Here's how the part is built. I have some questions about the finished solid (model axes, mm). A direction names the side the tool comes from. Give positions to 0.01 mm unless a question says otherwise; leave off trailing zeros. Loops run counter-clockwise (first coordinate to the right, second up) from the corner with the lowest first, then second, coordinate; pieces in that order, holes last.
Q1. Suppose I cut it at B-B (z = 27.5). List the corners of the cut face in (x, y) for me.
Q2. Suppose I cut it at D-D (y = -57). List the corners of the cut face in (x, z) for me.
Q3. I'm going to push flat-ended pins straight in: P1, Ø6, axis at x = 28.5, y = -5.5, coming from the -Z side; P2, Ø9, axis at y = 0, z = 0, coming from the -X side. Where does each tip first touch, or does it pass through?
Q4. For faces 5 (the face through (0, 7, 0)), 6 (the face through (5, 15, 0)), which set-ups out of +Z, -Z, +X, -X, +Y, -Y let a thin tool reach every point of the face, with its end or its side?
Q5. Suppose I cut it at A-A (y = 0). List the corners of the cut face in (x, z) for me.
Q6. I need wall thicknesses on probe 1 along X at (y, z) = (-14, -4); probe 2 along Y at (x, z) = (12.5, 0); probe 3 along Y at (x, z) = (38, 1.5). Which ranges of each line are inside material? Lowest first, please.
Q7. Suppose I cut it at C-C (x = 42.5). List the corners of the cut face in (y, z) for me, and give its area (3 significant figures).
Q8. Thinking about a two-plate mould opening in X: for faces 1 (the face through (2.535, 34.168, -7.587)), 2 (the face through (44.94, -57.14, -0.54)), 3 (the face through (22.745, 7.91, -10.316)), 4 (the face through (45, 7, 0)), which applies, pulls with the +X half, pulls with the -X half, needs draft (parallel to the pull), parting line crosses it, or undercut?
```python
from build123d import *

# Parameters (mm, degrees)
SKIZZE3_W = 2.5
SKIZZE3_H = 50


with BuildPart() as part:
    # Skizze1 → Rotation1 (revolve)
    with BuildSketch(Plane.XY, mode=Mode.PRIVATE) as rotation1_sk:
        Polygon((0, 5), (0, 35), (5, 35), (5, 13), (40, 13), (40, 35), (45, 35), (45, 5), align=None)
    revolve(rotation1_sk.sketch.rotate(Axis((-22.629795441, 0, 0), (1, 0, 0)), 90), axis=Axis((-22.629795441, 0, 0), (1, 0, 0)))  # turned: the seam where the file's is

    # Skizze3 → Rotation2 (revolve)
    with BuildSketch(Plane(origin=(42.5, 0, 0), x_dir=(0, 0, -1), z_dir=(1, 0, 0)), mode=Mode.PRIVATE) as rotation2_sk:
        with Locations((1.25, -55)):
            Rectangle(SKIZZE3_W, SKIZZE3_H)
    revolve(rotation2_sk.sketch.rotate(Axis((42.5, -30, 0), (0, -1, 0)), 180), axis=Axis((42.5, -30, 0), (0, -1, 0)))  # turned: the seam where the file's is


solid = part.part
```
Solutions:
1. outline: (0, -21.65) - (5, -21.65) - (5, 21.65) - (0, 21.65) - close; (40, -21.65) - (45, -21.65) - (45, 21.65) - (40, 21.65) - close
2. outline: circle Ø5 at (42.5, 0)
3. P1: stops at z = -12.76
3. P2: passes through
4. face 5: +Z, -Z, -X, +Y, -Y
4. face 6: none
5. outline: (0, -35) - (5, -35) - (5, -13) - (40, -13) - (40, -35) - (45, -35) - (45, -5) - (0, -5) - close; (0, 5) - (45, 5) - (45, 35) - (40, 35) - (40, 13) - (5, 13) - (5, 35) - (0, 35) - close
6. probe 1: x = 0 to 5, 40 to 45
6. probe 2: y = -13 to -5, 5 to 13
6. probe 3: y = -12.91 to -4.77, 4.77 to 12.91
7. outline: (-80, -2.5) - (-34.91, -2.5) arc R35 ccw (long way) to (-34.91, 2.5) - (-80, 2.5) - close; hole circle Ø10 at (0, 0)
7. area: 4,000 mm2
8. face 1: needs draft
8. face 2: parting line crosses it
8. face 3: undercut
8. face 4: pulls with the +X half
